Source: CAD feature listing. Evaluate the final solid. Frame: model axes, mm. A direction names the side the tool comes from. Coordinates: 2 decimals unless noted, no trailing zeros. Order: outer loops, then holes, each group sorted by start corner. A loop starts at its lowest first (then second) coordinate and runs counter-clockwise, first axis right, second up.
Solid Edge part; units mm, degrees
sketch "Sketch1" plane through (0, 0, 0) normal (0, -1, 0) x (1, 0, 0)
  line L0 (100.9821, -8.5934) -> (100.9821, 103.8022)
  arc A0 (97.1799, 107.6044) -> (100.9821, 103.8022) centre (97.1799, 103.8022) cw
  line L1 (97.1799, 107.6044) -> (-15.2157, 107.6044)
  arc A1 (-19.0179, 103.8022) -> (-15.2157, 107.6044) centre (-15.2157, 103.8022) cw
  line L2 (-19.0179, 103.8022) -> (-19.0179, -8.5934)
  arc A2 (-19.0179, -8.5934) -> (-15.2157, -12.3956) centre (-15.2157, -8.5934) ccw
  line L3 (-15.2157, -12.3956) -> (97.1799, -12.3956)
  arc A3 (100.9821, -8.5934) -> (97.1799, -12.3956) centre (97.1799, -8.5934) cw
extrude "Protrusion1" add sketch "Sketch1" along normal blind 40
sketch "Sketch2" plane through (0, 0, 0) normal (0, -1, 0) x (1, 0, 0)
  circle A0 centre (93.4821, -4.8956) radius 2.25
  circle A1 centre (-11.5179, -4.8956) radius 2.25
  circle A2 centre (-11.5179, 100.1044) radius 2.25
  circle A3 centre (93.4821, 100.1044) radius 2.25
extrude "Cutout1" cut sketch "Sketch2" along normal up to next
sketch "Sketch3" plane through (40.9821, -3.5, 47.6044) normal (0, 1, 0) x (-1, 0, 0)
  line L0 (-48.8101, 51.285) -> (-40.1098, 42.5847)
  arc A0 (-40.1098, 42.5847) -> (40.1098, 42.5847) centre (0, 0) cw
  line L1 (48.8101, 51.285) -> (40.1098, 42.5847)
  line L2 (50.0475, 50.0475) -> (48.8101, 51.285)
  line L3 (50.0475, 50.0475) -> (51.285, 48.8101)
  line L4 (51.285, 48.8101) -> (42.5847, 40.1098)
  arc A1 (42.5847, 40.1098) -> (42.5847, -40.1098) centre (0, 0) cw
  line L5 (51.285, -48.8101) -> (42.5847, -40.1098)
  line L6 (50.0475, -50.0475) -> (51.285, -48.8101)
  line L7 (50.0475, -50.0475) -> (48.8101, -51.285)
  line L8 (48.8101, -51.285) -> (40.1098, -42.5847)
  line L9 (-48.8101, -51.285) -> (-40.1098, -42.5847)
  line L10 (-50.0475, -50.0475) -> (-48.8101, -51.285)
  line L11 (-50.0475, -50.0475) -> (-51.285, -48.8101)
  line L12 (-51.285, -48.8101) -> (-42.5847, -40.1098)
  arc A2 (-42.5847, -40.1098) -> (-42.5847, 40.1098) centre (0, 0) cw
  line L13 (-51.285, 48.8101) -> (-42.5847, 40.1098)
  line L14 (-50.0475, 50.0475) -> (-51.285, 48.8101)
  line L15 (-50.0475, 50.0475) -> (-48.8101, 51.285)
  arc A3 (40.1098, -42.5847) -> (-40.1098, -42.5847) centre (0, 0) cw
  line L16 (60, 60) -> (-60, 60)
  line L17 (-60, 60) -> (-60, -60)
  line L18 (-60, -60) -> (60, -60)
  line L19 (60, -60) -> (60, 60)
extrude "拉伸除料_2" cut sketch "Sketch3" against normal blind 33
sketch "Sketch4" plane through (0, 0, 0) normal (0, -1, 0) x (1, 0, 0)
  circle A0 centre (40.9821, 47.6044) radius 57.5
extrude "拉伸除料_3" cut sketch "Sketch4" along normal blind 5
sketch "Sketch5" plane through (40.9821, -5, 47.6044) normal (0, 1, 0) x (1, 0, 0)
  circle A0 centre (0, 0) radius 31.5
  circle A1 centre (0, 0) radius 57.5
extrude "拉伸除料_4" cut sketch "Sketch5" against normal blind 20
sketch "Sketch6" plane through (40.9821, -25, 47.6044) normal (0, 1, 0) x (0, 0, 1)
  circle A0 centre (0, 0) radius 33.5
  circle A1 centre (0, 0) radius 57.5
extrude "拉伸除料_5" cut sketch "Sketch6" against normal blind 8
sketch "Sketch7" plane through (40.9821, -33, 47.6044) normal (0, 1, 0) x (0, 0, 1)
  line L0 (41.8772, -39.4024) -> (24.8932, -22.4183)
  arc A0 (41.8772, 39.4024) -> (41.8772, -39.4024) centre (0, 0) cw
  line L1 (41.8772, 39.4024) -> (24.8932, 22.4183)
  arc A1 (24.8932, 22.4183) -> (24.8932, -22.4183) centre (0, 0) cw
extrude "Cutout2" cut sketch "Sketch7" against normal up to next
sketch "Sketch8" plane through (40.9821, -33, 47.6044) normal (0, 1, 0) x (0, 0, 1)
  arc A0 (-39.4024, 41.8772) -> (39.4024, 41.8772) centre (0, 0) cw
  line L0 (39.4024, 41.8772) -> (22.4183, 24.8932)
  arc A1 (-22.4183, 24.8932) -> (22.4183, 24.8932) centre (0, 0) cw
  line L1 (-39.4024, 41.8772) -> (-22.4183, 24.8932)
extrude "Cutout3" cut sketch "Sketch8" against normal up to next
sketch "Sketch9" plane through (40.9821, -33, 47.6044) normal (0, 1, 0) x (0, 0, 1)
  line L0 (39.4024, -41.8772) -> (22.4183, -24.8932)
  arc A0 (22.4183, -24.8932) -> (-22.4183, -24.8932) centre (0, 0) cw
  line L1 (-39.4024, -41.8772) -> (-22.4183, -24.8932)
  arc A1 (39.4024, -41.8772) -> (-39.4024, -41.8772) centre (0, 0) cw
extrude "Cutout4" cut sketch "Sketch9" against normal up to next
sketch "Sketch10" plane through (40.9821, -33, 47.6044) normal (0, 1, 0) x (0, 0, 1)
  arc A0 (-24.8932, -22.4183) -> (-24.8932, 22.4183) centre (0, 0) cw
  line L0 (-41.8772, 39.4024) -> (-24.8932, 22.4183)
  line L1 (-41.8772, -39.4024) -> (-24.8932, -22.4183)
  arc A1 (-41.8772, -39.4023) -> (-41.8773, 39.4023) centre (0, 0) cw
extrude "Cutout5" cut sketch "Sketch10" against normal up to next
sketch "Sketch11" plane through (40.9821, -5, 47.6044) normal (0, 1, 0) x (1, 0, 0)
  circle A0 centre (0, 0) radius 2
extrude "拉伸除料_11" cut sketch "Sketch11" against normal blind 30
sketch "Sketch12" plane through (87.9169, -20, 92.0643) normal (0.7071, 0, -0.7071) x (0, -1, 0)
  circle A0 centre (-5.5, -2.152) radius 1.75
  circle A1 centre (5.5, -2.152) radius 1.75
extrude "Cutout6" cut sketch "Sketch12" against normal up to next
mirror "Mirror1" about plane through (40.9821, -38.25, 47.6044) normal (1, 0, 0) of "Cutout6"
mirror "Mirror2" about plane through (40.9821, -1.75, 47.6044) normal (0, 0, -1) of "Mirror1", "Cutout6"
1. Ray query, line 1 (Y direction, x = 96.5, z = 11); line 2 (Z direction, x = 49.5, y = -35); line 3 (X direction, y = -27.5, z = 78). Return the intervals inside material, ascending.
Findings:
line 1: y = -40 to -36.5, -3.5 to 0
line 2: z = -10.27 to -9.26, 15.21 to 80, 104.47 to 105.48
line 3: x = -9 to -7.83, 26.9 to 55.07, 89.79 to 90.97
2. Section query A-A on y = -31.5. Return loops of the section in (x, z).
Findings:
outline: (-10.3, -1.21) - (-9.07, -2.44) - (-7.83, -3.68) - (0.87, 5.02) arc R58.5 ccw to (81.09, 5.02) - (89.79, -3.68) - (91.03, -2.44) - (92.27, -1.21) - (83.57, 7.49) arc R58.5 ccw to (83.57, 87.71) - (92.27, 96.41) - (91.03, 97.65) - (89.79, 98.89) - (81.09, 90.19) arc R58.5 ccw to (0.87, 90.19) - (-7.83, 98.89) - (-9.07, 97.65) - (-10.3, 96.41) - (-1.6, 87.71) arc R58.5 ccw to (-1.6, 7.49) - close; circle Ø67 at (40.98, 47.6); hole circle Ø115 at (40.98, 47.6); hole circle Ø4 at (40.98, 47.6)
3. Section query D-D on y = -7.5. Return loops of the section in (x, z).
Findings:
outline: (-10.3, -1.21) - (-9.07, -2.44) - (-7.83, -3.68) - (0.87, 5.02) arc R58.5 ccw to (81.09, 5.02) - (89.79, -3.68) - (91.03, -2.44) - (92.27, -1.21) - (83.57, 7.49) arc R58.5 ccw to (83.57, 87.71) - (92.27, 96.41) - (91.03, 97.65) - (89.79, 98.89) - (81.09, 90.19) arc R58.5 ccw to (0.87, 90.19) - (-7.83, 98.89) - (-9.07, 97.65) - (-10.3, 96.41) - (-1.6, 87.71) arc R58.5 ccw to (-1.6, 7.49) - close; circle Ø63 at (40.98, 47.6); hole circle Ø115 at (40.98, 47.6); hole circle Ø4 at (40.98, 47.6)
4. Pin query (flat end, axial travel): P1, Ø15.5, axis at x = 13.5, z = 79.5, coming from the +Y side; P2, Ø1.5, axis at x = 76.5, y = -29, coming from the -Z side; P3, Ø7, axis at x = 93.48, z = 100.1, coming from the +Y side; P4, Ø8, axis at x = 42.5, z = 30, coming from the +Y side. Return the tip coordinate at first contact, or that it passes through.
Findings:
P1: stops at y = -33
P2: stops at z = 0.56
P3: stops at y = 0
P4: stops at y = -5
5. Access query for faces 1 (the face through (99.84, -38.23, 106.52)), 2 (the face through (32.4, -3.5, -10.5)), 3 (the face through (29, -25, 77)). Directions: +Z, -Z, +X, -X, +Y, -Y. A direction counts if a zero-diameter tool reaches every point of the face in a straight line with its end or side. Return the directions, or none.
Findings:
face 1: +Z, +X, +Y, -Y
face 2: none
face 3: +Y
6. Draft query along Y for faces 4 (the face through (9, -33, 80)), 5 (the face through (-6.014, -19.769, 92.125)), 6 (the face through (74.486, -36.451, 78.634)). Return one class per face: released by +Y, released by -Y, zero draft, split by the parting line, or undercut.
Findings:
face 4: released by +Y
face 5: undercut
face 6: zero draft
